The model under review builds one solid part; all positions refer to its coordinate system, in mm. Give positions to 0.01 mm unless a question says otherwise; leave off trailing zeros. Order: outer loops, then holes, each group sorted by start corner. A loop starts at its lowest first (then second) coordinate and runs counter-clockwise, first axis right, second up.
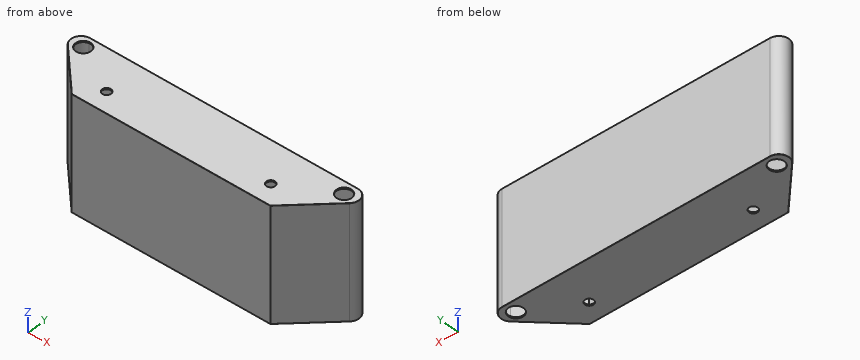
```python
from build123d import *

# Parameters (mm, degrees)
SKETCH1_W           = 460
SKETCH1_H           = 260
BOSS_EXTRUDE1_DEPTH = 3.04
BOSS_EXTRUDE2_DEPTH = 3.04
BOSS_EXTRUDE4_DEPTH = 260
FILLET1_R           = 0.5
SKETCH6_R           = 17.465
CUT_EXTRUDE1_DEPTH  = 444.976967296
SKETCH8_R           = 10
CUT_EXTRUDE2_DEPTH  = 444.976967296


with BuildPart() as part:
    # Sketch1 → Boss-Extrude1 (new body)
    with BuildSketch(Plane(origin=(0, 0, 0), x_dir=(1, 0, 0), z_dir=(0, 1, 0))):
        Rectangle(SKETCH1_W, SKETCH1_H)
    extrude(amount=BOSS_EXTRUDE1_DEPTH)

    # Sketch2 → Boss-Extrude2 (add)
    with BuildSketch(Plane.XY.offset(130)):
        with BuildLine():
            Line((-230, 0), (230, 0))
            Line((230, 0), (326.402020254, 96.402020254))
            ThreePointArc((326.402020254, 96.402020254), (331.430272212, 121.680749903), (310, 136))
            Line((310, 136), (-310, 136))
            ThreePointArc((-310, 136), (-331.430272212, 121.680749903), (-326.402020254, 96.402020254))
            Line((-326.402020254, 96.402020254), (-230, 0))
        make_face()
    boss_extrude2 = extrude(amount=-BOSS_EXTRUDE2_DEPTH)

    # Mirror1: Boss-Extrude2 across plane
    add(boss_extrude2.mirror(Plane.XY))

    # Sketch4 → Boss-Extrude4 (add)
    with BuildSketch(Plane(origin=(0, 0, -130), x_dir=(-1, 0, 0), z_dir=(0, 0, -1))):
        with BuildLine():
            Line((-326.402020254, 96.402020254), (-230, 0))
            Line((-230, 0), (230, 0))
            Line((230, 0), (326.402020254, 96.402020254))
            ThreePointArc((326.402020254, 96.402020254), (331.430272212, 121.680749903), (310, 136))
            Line((310, 136), (-310, 136))
            ThreePointArc((-310, 136), (-331.430272212, 121.680749903), (-326.402020254, 96.402020254))
        make_face()
        with BuildLine():
            Line((-324.252415639, 98.551624868), (-228.74079077, 3.04))
            Line((-228.74079077, 3.04), (228.74079077, 3.04))
            Line((228.74079077, 3.04), (324.252415639, 98.551624868))
            ThreePointArc((324.252415639, 98.551624868), (328.621678434, 120.517392268), (310, 132.96))
            Line((310, 132.96), (-310, 132.96))
            ThreePointArc((-310, 132.96), (-328.621678434, 120.517392268), (-324.252415639, 98.551624868))
        make_face(mode=Mode.SUBTRACT)
    extrude(amount=-BOSS_EXTRUDE4_DEPTH)

    # Fillet1
    fillet1_edges = [part.edges().sort_by_distance(p)[0] for p in [
        (278.201010127, 48.201010127, 130),
        (331.430272212, 121.680749903, 130),
        (0, 136, 130),
        (-331.430272212, 121.680749903, 130),
        (-278.201010127, 48.201010127, 130),
        (-278.201010127, 48.201010127, -130),
        (278.201010127, 48.201010127, -130),
        (331.430272212, 121.680749903, -130),
        (0, 136, -130),
        (-331.430272212, 121.680749903, -130),
        (0, 0, 130),
        (-230, 0, 0),
        (0, 0, -130),
        (230, 0, 0),
    ]]
    fillet(fillet1_edges, radius=FILLET1_R)

    # Sketch6 → Cut-Extrude1 (cut, through all)
    with BuildSketch(Plane(origin=(0, 0, -130), x_dir=(-1, 0, 0), z_dir=(0, 0, -1))):
        with Locations((-302.023340597, 109.5)):
            Circle(SKETCH6_R)
        with Locations((302.023340597, 109.5)):
            Circle(SKETCH6_R)
    extrude(amount=-CUT_EXTRUDE1_DEPTH, mode=Mode.SUBTRACT)

    # Sketch8 → Cut-Extrude2 (cut, through all)
    with BuildSketch(Plane.XY.offset(130)):
        with Locations((-190, 45.5)):
            Circle(SKETCH8_R)
        with Locations(Location((190, 45.5, 0), (0, 0, 180))):
            Circle(SKETCH8_R)
    extrude(amount=-CUT_EXTRUDE2_DEPTH, mode=Mode.SUBTRACT)


solid = part.part
```
Item 1: For line 1 (Y direction, x = 61, z = -101.5); line 2 (Z direction, x = 78.5, y = 19); line 3 (X direction, y = 54, z = -34.5), list the stretches that pass through material, from the lowest coordinate up.
Values found:
line 1: y = 0 to 3.04, 132.96 to 136
line 2: z = -130 to -126.96, 126.96 to 130
line 3: x = -284 to -279.7, 279.7 to 284
Item 2: Take a section at D-D (y = 109.5). Give the number of separate pieces and of enclosed holes in the cut face, and give its area (3 significant figures).
Values found:
separate pieces: 4
enclosed holes: 0
area: 5,190 mm2
Item 3: Clearance check with flat-ended pins moving along their axes: pin 1 Ø5 at (x, z) = (250, 11) entering from -Y; pin 2 Ø12 at (y, z) = (30.5, 46) entering from -X; pin 3 Ø1.5 at (y, z) = (62, 60.5) entering from -X. State where each tip first meets the part, or that it passes through.
Values found:
pin 1: stops at y = 17.5
pin 2: stops at x = -266.5
pin 3: stops at x = -292.75
Item 4: Take a section at A-A (x = -190). Give the boundary of the cut face in (y, z).
Values found:
outline: (0, -129.5) arc R0.5 ccw to (0.5, -130) - (35.5, -130) - (35.5, -126.96) - (3.04, -126.96) - (3.04, 126.96) - (35.5, 126.96) - (35.5, 130) - (0.5, 130) arc R0.5 ccw to (0, 129.5) - close; (55.5, -130) - (135.5, -130) arc R0.5 ccw to (136, -129.5) - (136, 129.5) arc R0.5 ccw to (135.5, 130) - (55.5, 130) - (55.5, 126.96) - (132.96, 126.96) - (132.96, -126.96) - (55.5, -126.96) - close
Item 5: Take a section at B-B (z = -58.5). Give the boundary of the cut face in (x, y), and give its area (3 significant figures).
Values found:
outline: (-326.4, 96.4) - (-230.15, 0.15) arc R0.5 ccw to (-229.79, 0) - (229.79, 0) arc R0.5 ccw to (230.15, 0.15) - (326.4, 96.4) arc R23.2 ccw to (310, 136) - (-310, 136) arc R23.2 ccw to start; hole (-324.25, 98.55) - (-228.74, 3.04) - (228.74, 3.04) - (324.25, 98.55) arc R20.16 ccw to (310, 132.96) - (-310, 132.96) arc R20.16 ccw to start
area: 4,410 mm2
Item 6: Take a section at C-C (x = 43). Give the boundary of the cut face in (y, z), and give its area (3 significant figures).
Values found:
outline: (0, -129.5) arc R0.5 ccw to (0.5, -130) - (135.5, -130) arc R0.5 ccw to (136, -129.5) - (136, 129.5) arc R0.5 ccw to (135.5, 130) - (0.5, 130) arc R0.5 ccw to (0, 129.5) - close; hole (3.04, -126.96) - (132.96, -126.96) - (132.96, 126.96) - (3.04, 126.96) - close
area: 2,370 mm2
